```python
from build123d import *

# Parameters (mm, degrees)
SKETCH5_R           = 1
BOSS_EXTRUDE2_DEPTH = 2
SKETCH8_R           = 1.315386289
BOSS_EXTRUDE4_DEPTH = 3
SKETCH11_W          = 1.206172966
SKETCH11_H          = 2
BOSS_EXTRUDE5_DEPTH = 7


with BuildPart() as part:
    # Sketch5 → Boss-Extrude2 (new body)
    with BuildSketch(Plane.XZ.offset(-9.339266183)):
        with Locations(Location((0, 0, 0), (0, 0, 270))):
            Circle(SKETCH5_R)
    extrude(amount=-BOSS_EXTRUDE2_DEPTH)

    # Sketch8 → Boss-Extrude4 (add)
    with BuildSketch(Plane(origin=(0, 11.339266183, 0), x_dir=(1, 0, 0), z_dir=(0, 1, 0))):
        with Locations(Location((0, 0, 0), (0, 0, 270))):
            Circle(SKETCH8_R)
    extrude(amount=BOSS_EXTRUDE4_DEPTH)

    # Sketch11 → Boss-Extrude5 (add)
    with BuildSketch(Plane(origin=(0, 0, 0), x_dir=(0, 0, -1), z_dir=(1, 0, 0))):
        with Locations((0, 12.810409413)):
            Rectangle(SKETCH11_W, SKETCH11_H)
    extrude(amount=-BOSS_EXTRUDE5_DEPTH)


solid = part.part
```
Check sheet for the modelled part. Datum: model origin and axes. Units: mm. A direction names the side the tool comes from. Coordinates: 2 decimals unless noted, no trailing zeros. Write each loop counter-clockwise with the first axis right and the second up, starting at its lowest first coordinate (ties: lowest second). Pieces come first, ordered by that corner, then holes. Notation, with made-up numbers: M -24.5,53 L -12.5,53 A12 cw -12.5,57 Z; hole C 73,73 d4. An arc over 180 degrees is marked long. Write item = value, one per line. Start each with the question number.
1. Sectioned sample at C-C (y = 10.15). Record the cut outline in (x, z).
2. Thickness scan on probe 1 along Y at (x, z) = (0.25, 1.2); probe 2 along Z at (x, y) = (-3, 12.9); probe 3 along Y at (x, z) = (-3, 0.4). Record the ranges inside material, lowest first.
3. Sectioned sample at B-B (z = 0). Record the cut outline in (x, y), then the cut area to 3 significant figures.
4. Sectioned sample at A-A (x = 0). Record the cut outline in (y, z), then the cut area to 3 significant figures.
5. Tool access check on faces 1 (the flat face through (0, 14.339, 0)), 2 (the flat face through (-4, 13, -0.603)), 3 (the cylindrical face through (-1, 10, 0)), 4 (the flat face through (-4, 13, 0.603)), 5 (the flat face through (-7, 13, 0)). Record the directions out of +Z, -Z, +X, -X, +Y, -Y that give a thin tool (end or side, any length) a straight path to the whole face; none if there is none.
6. Go/stop test with flat-tipped pins: pin 1 (1 mm diameter, centred on x = -4.5, y = 13, fed in from -Z); pin 2 (1 mm diameter, centred on x = -4.5, y = 13, fed in from +Z); pin 3 (0.6 mm diameter, centred on x = -5.5, z = 0, fed in from +Y). Record where each tip stops, or that it passes through.
7. Sectioned sample at D-D (x = -4.5). Record the cut outline in (y, z), then the cut area to 3 significant figures.
The answers:
q1.outline = C 0,0 d2
q2.probe_1 = 11.34 to 14.34
q2.probe_2 = -0.6 to 0.6
q2.probe_3 = 11.81 to 13.81
q3.outline = M -7,11.81 L -1.32,11.81 L -1.32,11.34 L -1,11.34 L -1,9.34 L 1,9.34 L 1,11.34 L 1.32,11.34 L 1.32,14.34 L -1.32,14.34 L -1.32,13.81 L -7,13.81 Z
q3.area = 23.3 mm²
q4.outline = M 9.34,-1 L 11.34,-1 L 11.34,-1.32 L 14.34,-1.32 L 14.34,1.32 L 11.34,1.32 L 11.34,1 L 9.34,1 Z
q4.area = 11.9 mm²
q5.face_1 = +Z, -Z, +X, -X, +Y
q5.face_2 = -Z, -X, +Y, -Y
q5.face_3 = -Y
q5.face_4 = +Z, -X, +Y, -Y
q5.face_5 = +Z, -Z, -X, +Y, -Y
q6.pin_1 = -0.6
q6.pin_2 = 0.6
q6.pin_3 = 13.81
q7.outline = M 11.81,-0.6 L 13.81,-0.6 L 13.81,0.6 L 11.81,0.6 Z
q7.area = 2.41 mm²
